CAD build for the part. Positions are in the model's coordinates, mm. A direction names the side the tool comes from. Give positions to 0.01 mm unless a question says otherwise; leave off trailing zeros. Loops run counter-clockwise (first coordinate to the right, second up) from the corner with the lowest first, then second, coordinate; pieces in that order, holes last.
Item 1: Which spindle directions (+Z, -Z, +X, -X, +Y, -Y) get a long thin tool onto all of the face, cutting with end or side? Do faces 1 (the flat face through (-24, 5, 27)), 2 (the flat face through (-17, 5, 40)), 3 (the flat face through (6, 7, 7)). Say none if no direction does.
Item 2: Saw through at C-C on y = 6.5. Give the cut face in (x, z), plus the area to 3 significant figures.
Item 3: Saw through at D-D on z = 5.5. Give the cut face in (x, y).
Item 4: Mould opens along X. For faces 4 (the cylindrical face through (8.483, 2.465, -0.26)), 5 (the flat face through (0, 5, 14)), 6 (the flat face through (8, 5, 2)) say: released by +X, released by -X, zero draft, split by the parting line, or undercut.
Item 5: Probe probe 1 along X at (y, z) = (1, 0); probe 2 along Z at (x, y) = (-13.5, 9); probe 3 along X at (y, z) = (1.75, 20). List the from-to ranges inside material, lowest first.
Item 6: Saw through at A-A on x = 6.5. Give the cut face in (y, z), plus the area to 4 significant figures.
Item 7: Drop flat-ended pins along their axis: P1, Ø6, axis at x = -37.5, y = 4, coming from the -Z side; P2, Ø5, axis at y = 6, z = 18, coming from the -X side; P3, Ø12, axis at x = -27, z = 27, coming from the -Y side; P4, Ø1.5, axis at y = 3, z = 31.5, coming from the -X side. Give the stop position or say it passes through.
Item 8: Saw through at B-B on y = 2.75. Give the cut face in (x, z).
from build123d import *

# Parameters (mm, degrees)
CROQUIS1_R              = 2
SALIENTE_EXTRUIR1_DEPTH = 10
CORTAR_EXTRUIR1_START   = -5
CROQUIS2_R              = 2
CORTAR_EXTRUIR1_DEPTH   = 5


with BuildPart() as part:
    # Croquis1 → Saliente-Extruir1 (new body)
    with BuildSketch(Plane(origin=(0, 0, 0), x_dir=(1, 0, 0), z_dir=(0, 1, 0))):
        with BuildLine():
            Line((13, 0), (13, -40))
            Line((13, -40), (-47, -40))
            ThreePointArc((-47, -40), (-53.5, -33.5), (-47, -27))
            Line((-47, -27), (0, -27))
            Line((0, -27), (0, 0))
            ThreePointArc((0, 0), (6.5, 6.5), (13, 0))
        make_face()
        with Locations(Location((6.5, 0, 0), (0, 0, 270))):
            Circle(CROQUIS1_R, mode=Mode.SUBTRACT)
    extrude(amount=SALIENTE_EXTRUIR1_DEPTH)

    # Croquis2 → Cortar-Extruir1 (cut)
    with BuildSketch(Plane(origin=(0, 10, 0), x_dir=(1, 0, 0), z_dir=(0, 1, 0)).offset(CORTAR_EXTRUIR1_START)):
        with BuildLine():
            Line((0, 0), (0, -7))
            Line((0, -7), (13, -7))
            Line((13, -7), (13, 0))
            ThreePointArc((13, 0), (6.5, 6.5), (0, 0))
        make_face()
        with Locations(Location((6.5, 0, 0), (0, 0, 270))):
            Circle(CROQUIS2_R, mode=Mode.SUBTRACT)
    extrude(amount=CORTAR_EXTRUIR1_DEPTH, mode=Mode.SUBTRACT)


solid = part.part
Results below:
1. face 1: -Z, -X, +Y, -Y
1. face 2: +Z, +X, -X, +Y, -Y
1. face 3: -Z, +X, -X, +Y
2. outline: (-47, 27) - (0, 27) - (0, 7) - (13, 7) - (13, 40) - (-47, 40) arc R6.5 ccw to start
2. area: 1,110 mm2
3. outline: (0, 0) - (13, 0) - (13, 5) - (0, 5) - close
4. face 4: undercut
4. face 5: released by -X
4. face 6: zero draft
5. probe 1: x = 0 to 4.5, 8.5 to 13
5. probe 2: z = 27 to 40
5. probe 3: x = 0 to 13
6. outline: (0, -6.5) - (5, -6.5) - (5, -2) - (0, -2) - close; (0, 2) - (5, 2) - (5, 7) - (10, 7) - (10, 40) - (0, 40) - close
6. area: 377.5 mm2
7. P1: stops at z = 27
7. P2: stops at x = 0
7. P3: stops at y = 0
7. P4: stops at x = -53.38
8. outline: (-47, 27) - (0, 27) - (0, 0) arc R6.5 ccw to (13, 0) - (13, 40) - (-47, 40) arc R6.5 ccw to start; hole circle Ø4 at (6.5, 0)
